Here's the drawing with two shaded views (mm, measured from the low corner). I have some questions. A direction names the side the tool comes from. Give positions to 0.01 mm unless a question says otherwise; leave off trailing zeros. Answer as a JSON object with one key per item and string values. Group by question number.
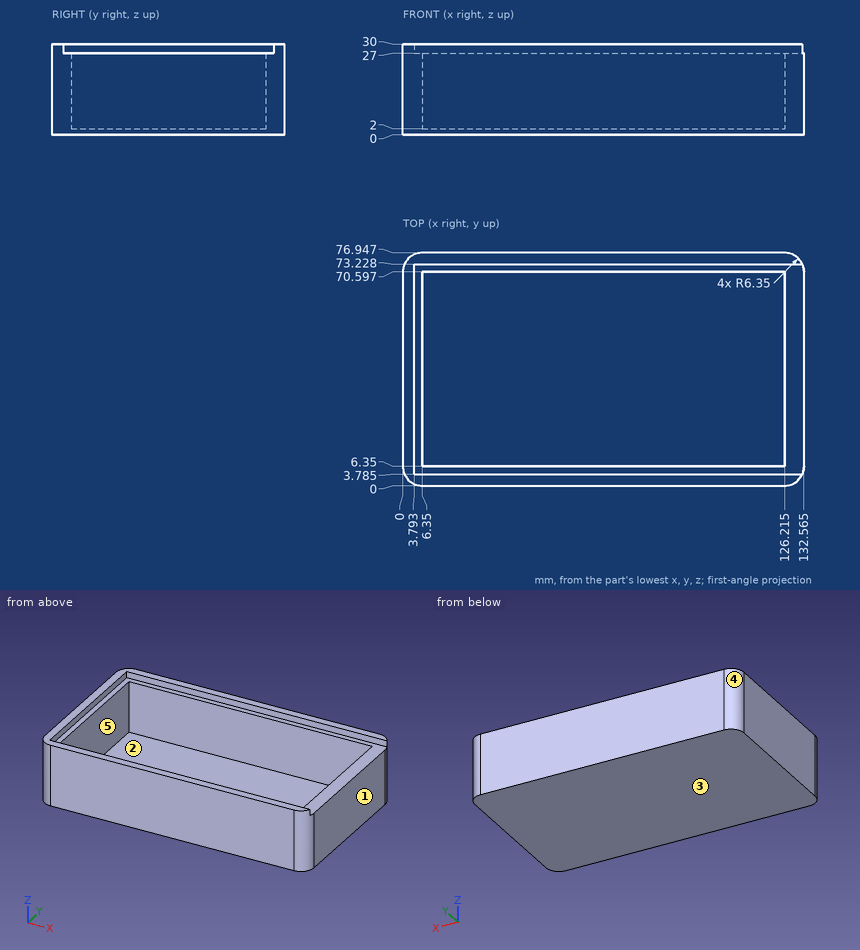
1) Please list where these lines run through material, in increasing order: line 1 along Y through (x, z) = (24, 23.75); line 2 along Y through (x, z) = (76, 28) (1 decimal); line 3 along Z through (x, y) = (16, 65.5). Write a range as from..to.
2) I'm going to push flat-ended pins straight in: pin 1 (5 mm diameter, centred on x = 105.5, y = 14.5, fed in from +Z); pin 2 (1.5 mm diameter, centred on y = 43.5, z = 28, fed in from +X). Where does each tip first touch, or does it pass through?
3) For the marked faces 1 and 2, which set-ups out of +Z, -Z, +X, -X, +Y, -Y let a thin tool reach every point of the face, with its end or its side?
4) We'd pull the mould along Y, two halves only. Please class the marked faces 3, 4 and 5: released by +Y, released by -Y, zero draft, split by the parting line, or undercut.
Taken from the geometry:
{
 "1": {"line 1": "0..6.35, 70.6..76.95", "line 2": "0..3.8, 73.2..76.9", "line 3": "0..2"},
 "2": {"pin 1": "z = 2", "pin 2": "x = 3.79"},
 "3": {"face 1": "+Z, -Z, +X, +Y, -Y", "face 2": "+Z"},
 "4": {"face 3": "zero draft", "face 4": "released by +Y", "face 5": "undercut"}
}
